The model under review builds one solid part; all positions refer to its coordinate system, in mm. A direction names the side the tool comes from. Coordinates: 2 decimals unless noted, no trailing zeros. Order: outer loops, then holes, each group sorted by start corner. A loop starts at its lowest first (then second) coordinate and runs counter-clockwise, first axis right, second up. Notation, with made-up numbers: (80, 11) -> (116, 11) arc R19 ccw to (116, 32) -> close; hole circle Ø11 at (47.5, 63). An arc over 180 degrees is marked (long way). Use one line per item in the form item = value.
from build123d import *

# Parameters (mm, degrees)
SKETCH1_R           = 15.875
BOSS_EXTRUDE1_DEPTH = 12.7


with BuildPart() as part:
    # Sketch1 → Boss-Extrude1 (new body)
    with BuildSketch(Plane.XY):
        with BuildLine():
            Line((17.434741505, 35.16914378), (23.951292477, 42.6577811))
            ThreePointArc((23.951292477, 42.6577811), (0, 95.25), (-23.951292477, 42.6577811))
            Line((-23.951292477, 42.6577811), (-17.434741505, 35.16914378))
            ThreePointArc((-17.434741505, 35.16914378), (-15.875741954, 31.097768382), (-17.309554442, 26.980638438))
            Line((-17.309554442, 26.980638438), (-23.594138681, 19.296295497))
            ThreePointArc((-23.594138681, 19.296295497), (0, -30.48), (23.594138681, 19.296295497))
            Line((23.594138681, 19.296295497), (17.309554442, 26.980638438))
            ThreePointArc((17.309554442, 26.980638438), (15.875741954, 31.097768382), (17.434741505, 35.16914378))
        make_face()
        with Locations((0, 63.5)):
            Circle(SKETCH1_R, mode=Mode.SUBTRACT)
        Circle(SKETCH1_R, mode=Mode.SUBTRACT)
    extrude(amount=BOSS_EXTRUDE1_DEPTH)


solid = part.part
Item 1: Draft analysis for pull direction X (two halves, no side actions). For faces 1 (the face through (-0.963, -30.465, 6.261)), 2 (the face through (-3.441, -15.497, 6.261)), 3 (the face through (20.5, 23.08, 6.26)), 4 (the face through (0, 33, 0)), state which applies: released by +X, released by -X, zero draft, split by the parting line, or undercut.
Results found:
face_1 = split by the parting line
face_2 = undercut
face_3 = released by +X
face_4 = zero draft
Item 2: We need section A-A (y = 63.5). Write out the cut boundary in (x, z) (3 decimals), plus the area to 3 significant figures.
Results found:
outline = (-31.75, 0) -> (-15.875, 0) -> (-15.875, 12.7) -> (-31.75, 12.7) -> close; (15.875, 0) -> (31.75, 0) -> (31.75, 12.7) -> (15.875, 12.7) -> close
area = 403 mm²
Item 3: Clearance check with flat-ended pins moving along their axes: pin 1 (6 mm diameter, centred on x = -17, z = 9.5, fed in from -Y); pin 2 (1 mm diameter, centred on x = 14.5, y = 38, fed in from -Z); pin 3 (6 mm diameter, centred on x = -7.5, z = 5, fed in from +Y). State where each tip first meets the part, or that it passes through.
Results found:
pin_1 = -27.07
pin_2 = 0
pin_3 = 94.93
Item 4: Tool access review of faces 5 (the face through (1.016, 95.234, 6.261)), 6 (the face through (20.647, 38.861, 6.261)), 7 (the face through (-20.74, 38.97, 6.26)): name each direction out of +Z, -Z, +X, -X, +Y, -Y from which nothing blocks a thin tool from reaching the whole face with its end or side.
Results found:
face_5 = +Z, -Z
face_6 = +Z, -Z, +X
face_7 = +Z, -Z, -X
Item 5: We need section B-B (x = 0). Write out the cut boundary in (y, z) (3 decimals).
Results found:
outline = (-30.48, 0) -> (-15.875, 0) -> (-15.875, 12.7) -> (-30.48, 12.7) -> close; (15.875, 0) -> (47.625, 0) -> (47.625, 12.7) -> (15.875, 12.7) -> close; (79.375, 0) -> (95.25, 0) -> (95.25, 12.7) -> (79.375, 12.7) -> close
Item 6: We need section C-C (z = 11.25). Write out the cut boundary in (x, y) (3 decimals).
Results found:
outline = (-23.951, 42.658) -> (-17.435, 35.169) arc R6.35 cw to (-17.31, 26.981) -> (-23.594, 19.296) arc R30.48 ccw (long way) to (23.594, 19.296) -> (17.31, 26.981) arc R6.35 cw to (17.435, 35.169) -> (23.951, 42.658) arc R31.75 ccw (long way) to start; hole circle Ø31.75 at (0, 0); hole circle Ø31.75 at (0, 63.5)
Item 7: We need section D-D (x = -28). Write out the cut boundary in (y, z), plus the area to 3 significant figures.
Results found:
outline = (-12.04, 0) -> (12.04, 0) -> (12.04, 12.7) -> (-12.04, 12.7) -> close; (48.53, 0) -> (78.47, 0) -> (78.47, 12.7) -> (48.53, 12.7) -> close
area = 686 mm²
Item 8: To check wall thickness, follow L1, parallel to Y at x = 0, z = 9.5 (3 decimals); L2, parallel to Y at x = -9.5, z = 5.25; L3, parallel to X at y = 63, z = 11. State the ranges of each line that lie inside material, in increasing order. Write a range as from..to.
Results found:
L1 = -30.48..-15.875, 15.875..47.625, 79.375..95.25
L2 = -28.96..-12.72, 12.72..50.78, 76.22..93.8
L3 = -31.75..-15.87, 15.87..31.75
